Verification items for the finished model (mm, model axes). Face numbers are marked on the shaded views. A direction names the side the tool comes from. Give positions to 0.01 mm unless a question says otherwise; leave off trailing zeros. Order: outer loops, then holes, each group sorted by start corner. A loop starts at its lowest first (then second) coordinate and runs counter-clockwise, first axis right, second up.
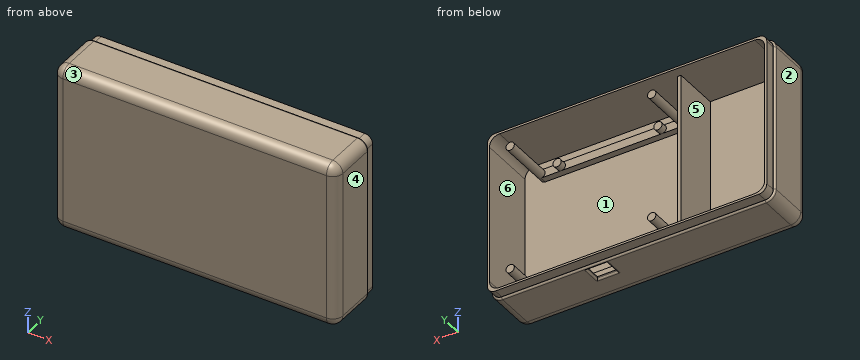
from build123d import *

# Parameters (mm, degrees)
SKETCH2_W           = 54.5
SKETCH2_H           = 47.5
SKETCH2_W_2         = 1
SKETCH2_W_3         = 27
BOSS_EXTRUDE3_DEPTH = 1.25
SKETCH2_4_W         = 85
SKETCH2_4_H         = 50
SKETCH2_4_W_2       = 82.5
SKETCH2_4_H_2       = 47.5
BOSS_EXTRUDE4_DEPTH = 18
SKETCH2_5_W         = 1
SKETCH2_5_H         = 47.5
BOSS_EXTRUDE5_DEPTH = 15
SKETCH5_R           = 1.2446
BOSS_EXTRUDE6_DEPTH = 16.5
SKETCH6_R           = 1.2446
BOSS_EXTRUDE7_DEPTH = 4
SKETCH7_W           = 42.418
SKETCH7_H           = 2.4892
BOSS_EXTRUDE9_DEPTH = 2
FILLET2_R           = 3
SKETCH10_OUTSIDE_W  = 107.048
SKETCH10_OUTSIDE_H  = 72.048
CUT_EXTRUDE4_DEPTH  = 3
FILLET3_R           = 0.5
SKETCH14_W          = 6
SKETCH14_H          = 5
CUT_EXTRUDE5_DEPTH  = 2
FILLET4_R           = 0.5


with BuildPart() as part:
    # Sketch2 → Boss-Extrude3 (new body)
    with BuildSketch(Plane(origin=(0, 0, 0), x_dir=(1, 0, 0), z_dir=(0, 1, 0))):
        with Locations((14, 0)):
            Rectangle(SKETCH2_W, SKETCH2_H)
        with Locations((-13.75, 0)):
            Rectangle(SKETCH2_W_2, SKETCH2_H)
        with Locations((-27.75, 0)):
            Rectangle(SKETCH2_W_3, SKETCH2_H)
    extrude(amount=BOSS_EXTRUDE3_DEPTH)

    # Sketch2<4> → Boss-Extrude4 (add)
    with BuildSketch(Plane(origin=(0, 0, 0), x_dir=(1, 0, 0), z_dir=(0, 1, 0))):
        Rectangle(SKETCH2_4_W, SKETCH2_4_H)
        Rectangle(SKETCH2_4_W_2, SKETCH2_4_H_2, mode=Mode.SUBTRACT)
    extrude(amount=BOSS_EXTRUDE4_DEPTH)

    # Sketch2<5> → Boss-Extrude5 (add)
    with BuildSketch(Plane(origin=(0, 0, 0), x_dir=(1, 0, 0), z_dir=(0, 1, 0))):
        with Locations((-13.75, 0)):
            Rectangle(SKETCH2_5_W, SKETCH2_5_H)
    extrude(amount=BOSS_EXTRUDE5_DEPTH)

    # Sketch5 → Boss-Extrude6 (add)
    with BuildSketch(Plane(origin=(0, 1.25, 0), x_dir=(1, 0, 0), z_dir=(0, 1, 0))):
        with Locations(Location((-7.209, 18.923, 0), (0, 0, 270))):
            Circle(SKETCH5_R)
        with Locations(Location((35.209, 18.923, 0), (0, 0, 270))):
            Circle(SKETCH5_R)
        with Locations(Location((-7.209, -18.923, 0), (0, 0, 270))):
            Circle(SKETCH5_R)
        with Locations(Location((35.209, -18.923, 0), (0, 0, 270))):
            Circle(SKETCH5_R)
    extrude(amount=BOSS_EXTRUDE6_DEPTH)

    # Sketch6 → Boss-Extrude7 (add)
    with BuildSketch(Plane(origin=(0, 1.25, 0), x_dir=(1, 0, 0), z_dir=(0, 1, 0))):
        with Locations(Location((-1.113, 18.923, 0), (0, 0, 270))):
            Circle(SKETCH6_R)
        with Locations(Location((29.113, 18.923, 0), (0, 0, 270))):
            Circle(SKETCH6_R)
        with Locations(Location((-1.113, -18.923, 0), (0, 0, 270))):
            Circle(SKETCH6_R)
        with Locations(Location((29.113, -18.923, 0), (0, 0, 270))):
            Circle(SKETCH6_R)
    extrude(amount=BOSS_EXTRUDE7_DEPTH)

    # Sketch7 → Boss-Extrude9 (add)
    with BuildSketch(Plane(origin=(0, 1.25, 0), x_dir=(1, 0, 0), z_dir=(0, 1, 0))):
        with Locations((14, -18.923)):
            Rectangle(SKETCH7_W, SKETCH7_H)
        with Locations((14, 18.923)):
            Rectangle(SKETCH7_W, SKETCH7_H)
    extrude(amount=BOSS_EXTRUDE9_DEPTH)

    # Fillet2
    fillet2_edges = [part.edges().sort_by_distance(p)[0] for p in [
        (41.25, 9.625, 23.75),
        (-41.25, 9.625, 23.75),
        (-41.25, 9.625, -23.75),
        (0, 0, 25),
        (-42.5, 9, 25),
        (42.5, 0, 0),
        (42.5, 9, 25),
        (42.5, 9, -25),
        (-42.5, 9, -25),
        (41.25, 9.625, -23.75),
        (-42.5, 0, 0),
        (0, 0, -25),
    ]]
    fillet(fillet2_edges, radius=FILLET2_R)

    # Sketch10 outside → Cut-Extrude4 (cut)
    with BuildSketch(Plane(origin=(0, 18, 0), x_dir=(1, 0, 0), z_dir=(0, 1, 0))):
        Rectangle(SKETCH10_OUTSIDE_W, SKETCH10_OUTSIDE_H)
        with BuildLine():
            Line((-41.875, 22), (-41.875, -22))
            ThreePointArc((-41.875, -22), (-41.179378605, -23.679378605), (-39.5, -24.375))
            Line((-39.5, -24.375), (39.5, -24.375))
            ThreePointArc((39.5, -24.375), (41.179378605, -23.679378605), (41.875, -22))
            Line((41.875, -22), (41.875, 22))
            ThreePointArc((41.875, 22), (41.179378605, 23.679378605), (39.5, 24.375))
            Line((39.5, 24.375), (-39.5, 24.375))
            ThreePointArc((-39.5, 24.375), (-41.179378605, 23.679378605), (-41.875, 22))
        make_face(mode=Mode.SUBTRACT)
    extrude(amount=-CUT_EXTRUDE4_DEPTH, mode=Mode.SUBTRACT)

    # Fillet3
    fillet3_edges = [part.edges().sort_by_distance(p)[0] for p in [
        (41.621320344, 15, -24.121320344),
        (0, 15, 25),
        (42.5, 15, 0),
        (-41.621320344, 15, 24.121320344),
        (-42.5, 15, 0),
        (-41.621320344, 15, -24.121320344),
        (0, 15, -25),
        (41.621320344, 15, 24.121320344),
    ]]
    fillet(fillet3_edges, radius=FILLET3_R)

    # Sketch14 → Cut-Extrude5 (cut)
    with BuildSketch(Plane.XY.offset(-25)):
        with Locations((11.587, 11.5)):
            Rectangle(SKETCH14_W, SKETCH14_H)
    extrude(amount=CUT_EXTRUDE5_DEPTH, mode=Mode.SUBTRACT)

    # Fillet4
    fillet4_edges = [part.edges().sort_by_distance(p)[0] for p in [
        (8.587, 11.5, -23.75),
        (11.587, 9, -23.75),
        (14.587, 11.5, -25),
        (11.587, 14, -25),
        (14.587, 11.5, -23.75),
        (11.587, 14, -23.75),
        (8.587, 11.5, -25),
        (11.587, 9, -25),
    ]]
    fillet(fillet4_edges, radius=FILLET4_R - 0.0001)  # a hair under: the kernel refuses the full size


solid = part.part
(1) Scan lines: line 1 (X direction, y = 9, z = 2); line 2 (Z direction, x = -1, y = 3.75); line 3 (Z direction, x = 5, y = 12). Record each from-to range of solid material in increasing order.
Solved:
line 1: x = -42.5 to -41.25, -14.25 to -13.25, 41.25 to 42.5
line 2: z = -25 to -23.75, -20.16 to -17.68, 17.68 to 20.16, 23.75 to 25
line 3: z = -25 to -23.75, 23.75 to 25
(2) Set-up check for the marked faces 1 and 2: record each of +Z, -Z, +X, -X, +Y, -Y from which the full face is reachable in a straight line by a thin tool's end or side.
Solved:
face 1: +Y
face 2: +Z, -Z, -X, +Y, -Y
(3) Section check D-D, the plane x = 25.5. Enter the section's corners in (y, z) (3 decimals), then the cut area to 3 significant figures.
Solved:
outline: (0, -22) arc R3 ccw to (3, -25) - (14.5, -25) arc R0.5 ccw to (15, -24.5) - (15, -24.375) - (18, -24.375) - (18, -23.75) - (1.25, -23.75) - (1.25, -20.168) - (3.25, -20.168) - (3.25, -17.678) - (1.25, -17.678) - (1.25, 17.678) - (3.25, 17.678) - (3.25, 20.168) - (1.25, 20.168) - (1.25, 23.75) - (18, 23.75) - (18, 24.375) - (15, 24.375) - (15, 24.5) arc R0.5 ccw to (14.5, 25) - (3, 25) arc R3 ccw to (0, 22) - close
area: 107 mm2
(4) Section check A-A, the plane y = 4.25. Give the number of separate pieces and of enclosed holes in the cut face, then the cut area to 3 significant figures.
Solved:
separate pieces: 9
enclosed holes: 2
area: 418 mm2
(5) Go/stop test with flat-tipped pins: pin 1 (2 mm diameter, centred on x = 35, z = 18.5, fed in from +Y); pin 2 (4 mm diameter, centred on x = 30.5, z = -19.5, fed in from +Y); pin 3 (0.6 mm diameter, centred on x = 18, y = 2, fed in from +Z). Record where each tip stops, or that it passes through.
Solved:
pin 1: stops at y = 17.75
pin 2: stops at y = 5.25
pin 3: stops at z = 24.92
(6) Release check for a two-part mould opening along X. For the marked faces 3, 4, 5 and 6 record: pulls with the +X half, pulls with the -X half, needs draft (parallel to the pull), parting line crosses it, or undercut.
Solved:
face 3: needs draft
face 4: pulls with the +X half
face 5: undercut
face 6: undercut
(7) Section check C-C, the plane z = -11. Enter the section's corners in (x, y) (3 decimals).
Solved:
outline: (-42.5, 3) arc R3 ccw to (-39.5, 0) - (39.5, 0) arc R3 ccw to (42.5, 3) - (42.5, 14.5) arc R0.5 ccw to (42, 15) - (41.875, 15) - (41.875, 18) - (41.25, 18) - (41.25, 1.25) - (-13.25, 1.25) - (-13.25, 15) - (-14.25, 15) - (-14.25, 1.25) - (-41.25, 1.25) - (-41.25, 18) - (-41.875, 18) - (-41.875, 15) - (-42, 15) arc R0.5 ccw to (-42.5, 14.5) - close
